Geometry: final body of the model. Coordinates: model frame, mm. Give positions to 0.01 mm unless a question says otherwise; leave off trailing zeros. Write each loop counter-clockwise with the first axis right and the second up, starting at its lowest first coordinate (ties: lowest second). Pieces come first, ordered by that corner, then holes. Notation, with made-up numbers: M -33.5,-25.5 L -24.5,-25.5 A27 cw -24.5,11.5 Z; hole C 87,78.25 d4. An arc over 180 degrees is marked long. Use a Markdown table: item, result. Add a question column.
1) Section A-A on z = 184. Return the cut outline in (x, y), then the cut area to 3 significant figures.
2) Line query: line 1 (Y direction, x = -3.25, z = 133); line 2 (X direction, y = -1.7, z = 255); line 3 (X direction, y = 1.5, z = 111). Output: solid intervals per line, ascending.
3) Pin query (flat end, axial travel): pin 1 (4.5 mm diameter, centred on x = 0, z = 315, fed in from +Y); pin 2 (1.8 mm diameter, centred on x = -0.5, z = 114.5, fed in from +Y). Return the tip coordinate at first contact, or that it passes through.
```python
from build123d import *

# Parameters (mm, degrees)
EXTRUDE1_DEPTH             = 600
EXTRUDE2_REACH             = 602.052
SKETCH2_R                  = 1.75
SKETCH_R                   = 3
SKETCH_R_2                 = 1.75
EXTRUDE4_DEPTH             = 3.5
CHAMFER1_SIZE              = 0.2
LPATTERN1_COUNT            = 30
LPATTERN1_PITCH            = 20
CHAMFER1_OF_LPATTERN1_SIZE = 0.2


with BuildPart() as part:
    # Sketch1 → Extrude1 (new body)
    with BuildSketch(Plane.XY):
        with BuildLine():
            Line((-4.3, -3.25), (4.3, -3.25))
            Line((4.3, -3.25), (4.5, -3.05))
            Line((4.5, -3.05), (4.5, 0.455012563))
            ThreePointArc((4.5, 0.455012563), (3.924845827, 0.712323349), (3.617735397, 1.2625))
            Line((3.617735397, 1.2625), (3.15008224, 1.2625))
            Line((3.15008224, 1.2625), (3.15008224, 1.7625))
            Line((3.15008224, 1.7625), (3.65008224, 1.7625))
            ThreePointArc((3.65008224, 1.7625), (3.973877727, 2.229724887), (4.5, 2.444987437))
            Line((4.5, 2.444987437), (4.5, 3.05))
            Line((4.5, 3.05), (4.3, 3.25))
            Line((4.3, 3.25), (-4.3, 3.25))
            Line((-4.3, 3.25), (-4.5, 3.05))
            Line((-4.5, 3.05), (-4.5, 2.444987437))
            ThreePointArc((-4.5, 2.444987437), (-3.973877727, 2.229724887), (-3.65008224, 1.7625))
            Line((-3.65008224, 1.7625), (-3.15008224, 1.7625))
            Line((-3.15008224, 1.7625), (-3.15008224, 1.2625))
            Line((-3.15008224, 1.2625), (-3.617735397, 1.2625))
            ThreePointArc((-3.617735397, 1.2625), (-3.924845827, 0.712323349), (-4.5, 0.455012563))
            Line((-4.5, 0.455012563), (-4.5, -3.05))
            Line((-4.5, -3.05), (-4.3, -3.25))
        make_face()
    extrude(amount=EXTRUDE1_DEPTH)

    # Sketch2 → Extrude2 (cut, up to next)
    with BuildSketch(Plane(origin=(0, 3.25, 0), x_dir=(1, 0, 0), z_dir=(0, 1, 0)), mode=Mode.PRIVATE) as extrude2_sk1:
        with Locations(Location((0, -15, 0), (0, 0, 270))):
            Circle(SKETCH2_R)
    extrude2_tool1 = extrude(extrude2_sk1.sketch, amount=-EXTRUDE2_REACH, mode=Mode.PRIVATE) & part.part
    extrude2 = extrude2_tool1.solids().sort_by_distance((0, 3.25, 15))[0]
    add(extrude2, mode=Mode.SUBTRACT)

    # Sketch → Extrude4 (cut)
    with BuildSketch(Plane(origin=(0, 3.25, 0), x_dir=(1, 0, 0), z_dir=(0, 1, 0))):
        with Locations(Location((0, -15, 0), (0, 0, 270))):
            Circle(SKETCH_R)
        with Locations(Location((0, -15, 0), (0, 0, 270))):
            Circle(SKETCH_R_2, mode=Mode.SUBTRACT)
    extrude4 = extrude(amount=-EXTRUDE4_DEPTH, mode=Mode.SUBTRACT)

    # Chamfer1
    chamfer1_edges = [part.edges().sort_by_distance(p)[0] for p in [
        (0, -3.25, 13.25),
        (0, 3.25, 12),
    ]]
    chamfer(chamfer1_edges, length=CHAMFER1_SIZE)

    # LPattern1: Extrude2, Extrude4 ×30
    with Locations(*[(0, 0, i * LPATTERN1_PITCH) for i in range(1, LPATTERN1_COUNT)]):
        add(extrude2, mode=Mode.SUBTRACT)
        add(extrude4, mode=Mode.SUBTRACT)

    # Chamfer1 of LPattern1
    chamfer1_of_lpattern1_edges = [part.edges().sort_by_distance(p)[0] for p in [
        (0, -3.25, 33.25),
        (0, 3.25, 32),
        (0, -3.25, 53.25),
        (0, 3.25, 52),
        (0, -3.25, 73.25),
        (0, 3.25, 72),
        (0, -3.25, 93.25),
        (0, 3.25, 92),
        (0, -3.25, 113.25),
        (0, 3.25, 112),
        (0, -3.25, 133.25),
        (0, 3.25, 132),
        (0, -3.25, 153.25),
        (0, 3.25, 152),
        (0, -3.25, 173.25),
        (0, 3.25, 172),
        (0, -3.25, 193.25),
        (0, 3.25, 192),
        (0, -3.25, 213.25),
        (0, 3.25, 212),
        (0, -3.25, 233.25),
        (0, 3.25, 232),
        (0, -3.25, 253.25),
        (0, 3.25, 252),
        (0, -3.25, 273.25),
        (0, 3.25, 272),
        (0, -3.25, 293.25),
        (0, 3.25, 292),
        (0, -3.25, 313.25),
        (0, 3.25, 312),
        (0, -3.25, 333.25),
        (0, 3.25, 332),
        (0, -3.25, 353.25),
        (0, 3.25, 352),
        (0, -3.25, 373.25),
        (0, 3.25, 372),
        (0, -3.25, 393.25),
        (0, 3.25, 392),
        (0, -3.25, 413.25),
        (0, 3.25, 412),
        (0, -3.25, 433.25),
        (0, 3.25, 432),
        (0, -3.25, 453.25),
        (0, 3.25, 452),
        (0, -3.25, 473.25),
        (0, 3.25, 472),
        (0, -3.25, 493.25),
        (0, 3.25, 492),
        (0, -3.25, 513.25),
        (0, 3.25, 512),
        (0, -3.25, 533.25),
        (0, 3.25, 532),
        (0, -3.25, 553.25),
        (0, 3.25, 552),
        (0, -3.25, 573.25),
        (0, 3.25, 572),
        (0, -3.25, 593.25),
        (0, 3.25, 592),
    ]]
    chamfer(chamfer1_of_lpattern1_edges, length=CHAMFER1_OF_LPATTERN1_SIZE)


solid = part.part
```
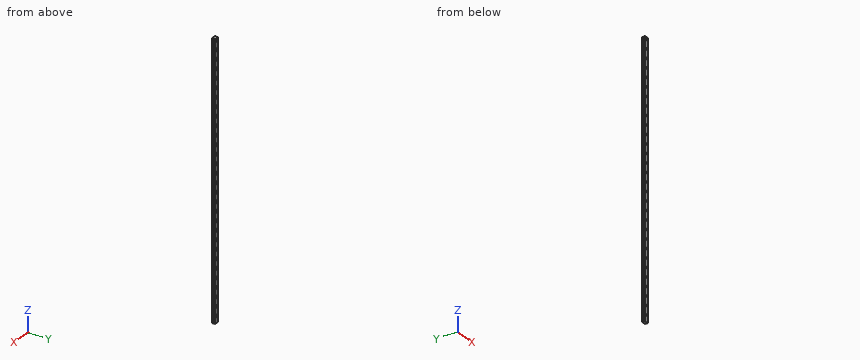
Found:
| question | item | result |
|---|---|---|
| 1 | outline | M -4.5,-3.05 L -4.3,-3.25 L 4.3,-3.25 L 4.5,-3.05 L 4.5,0.46 A1 cw 3.62,1.26 L 3.15,1.26 L 3.15,1.76 L 3.65,1.76 A1 cw 4.5,2.44 L 4.5,3.05 L 4.3,3.25 L -4.3,3.25 L -4.5,3.05 L -4.5,2.44 A1 cw -3.65,1.76 L -3.15,1.76 L -3.15,1.26 L -3.62,1.26 A1 cw -4.5,0.46 Z |
| 1 | area | 55.2 mm² |
| 2 | line 1 | -3.25 to 1.26, 1.76 to 3.25 |
| 2 | line 2 | -4.5 to -1.75, 1.75 to 4.5 |
| 2 | line 3 | -3.15 to 3.15 |
| 3 | pin 1 | y = -0.25 |
| 3 | pin 2 | through |
